The model under review builds one solid part; all positions refer to its coordinate system, in mm. A direction names the side the tool comes from. Give positions to 0.01 mm unless a question says otherwise; leave off trailing zeros. Loops run counter-clockwise (first coordinate to the right, second up) from the corner with the lowest first, then second, coordinate; pieces in that order, holes last. Notation, with made-up numbers: M 17,-33 L 50,-33 A37 cw 50,5 Z; hole C 2,17 d1. An arc over 180 degrees is marked long. One line per item, written item: value. Start each with the question number.
Q1. Mouldability with a two-part tool opening along Y and no side actions: class faces 1 (the face through (-1, 12.5, 3)), 2 (the face through (-56.426, 3.745, 2.958)), 3 (the face through (-32.022, 0.466, 2.958)), 4 (the face through (1, 0, 6)) as released by +Y, released by -Y, zero draft, split by the parting line, or undercut.
Q2. We need section C-C on z = 1. Give the number of separate pieces and of enclosed holes in the cut face, plus the area to 3 significant figures.
Q3. For faces 5 (the face through (16.928, -4.484, 2.958)), 6 (the face through (-37, -7, 3)), 7 (the face through (-33, -10, 3)), list the 3-axis set-ups (+Z, -Z, +X, -X, +Y, -Y) from which the entire face can be reached by the end or side of a thin tool; tool diameter is ignored.
Q4. We need section B-B on y = 0. Write out the cut boundary in (x, z).
Q5. For pin 1 (3.5 mm diameter, centred on x = -35.5, y = -6, fed in from -Z); pin 2 (3 mm diameter, centred on x = -30, z = 3, fed in from -Y); pin 3 (3 mm diameter, centred on y = 5, z = 2.5, fed in from +X), all flat-tipped, find the tip position at first contact; note any pin that passes through.
Q6. We need section D-D on x = -43.5. Write out the cut boundary in (y, z), plus the area to 3 significant figures.
Q7. We need section A-A on x = -5.5. Write out the cut boundary in (y, z).
Q8. To check wall thickness, follow line 1 along X through (y, z) = (5, 5.05); line 2 along X through (y, z) = (-1.75, 0.65); line 3 along Y through (x, z) = (-35.5, 4.75). State the ranges of each line that lie inside material, in increasing order. Write a range as from..to.
```python
from build123d import *

# Parameters (mm, degrees)
SKETCH1_R                                       = 4
SKETCH1_R_2                                     = 1.55
SKETCH1_R_3                                     = 7.5
BOSS_EXTRUDE1_DEPTH                             = 6
CSK_FOR_M5_FLAT_HEAD_MACHINE_SCREW1_D           = 5.5
CSK_FOR_M5_FLAT_HEAD_MACHINE_SCREW1_CSINK_D     = 10.4
CSK_FOR_M5_FLAT_HEAD_MACHINE_SCREW1_CSINK_ANGLE = 90
SKETCH4_R                                       = 1.55
SKETCH4_R_2                                     = 7.5
CUT_EXTRUDE1_DEPTH                              = 59.662168388
SKETCH6_R                                       = 3
CUT_EXTRUDE3_DEPTH                              = 3


with BuildPart() as part:
    # Sketch1 → Boss-Extrude1 (new body)
    with BuildSketch(Plane.XY):
        with BuildLine():
            Line((-44.5, 12.5), (44.5, 12.5))
            ThreePointArc((44.5, 12.5), (57, 0), (44.5, -12.5))
            Line((44.5, -12.5), (-12, -12.5))
            Line((-12, -12.5), (-14.5, -10))
            Line((-14.5, -10), (-52, -10))
            ThreePointArc((-52, -10), (-56.358541226, 3.952847075), (-44.5, 12.5))
        make_face()
        with Locations((10.5, 0)):
            Circle(SKETCH1_R, mode=Mode.SUBTRACT)
        with Locations((15.449747468, 4.949747468)):
            Circle(SKETCH1_R_2, mode=Mode.SUBTRACT)
        with Locations(Location((5.550252532, 4.949747468, 0), (0, 0, 180))):
            Circle(SKETCH1_R_2, mode=Mode.SUBTRACT)
        with Locations((5.550252532, -4.949747468)):
            Circle(SKETCH1_R_2, mode=Mode.SUBTRACT)
        with Locations((15.449747468, -4.949747468)):
            Circle(SKETCH1_R_2, mode=Mode.SUBTRACT)
        with Locations((-33.5, 0)):
            Circle(SKETCH1_R_2, mode=Mode.SUBTRACT)
        with Locations((-19.5, 0)):
            Circle(SKETCH1_R_3, mode=Mode.SUBTRACT)
        with Locations((-5.5, 0)):
            Circle(SKETCH1_R_2, mode=Mode.SUBTRACT)
    extrude(amount=BOSS_EXTRUDE1_DEPTH)

    # CSK for M5 Flat Head Machine Screw1 (through all)
    with Locations(Plane.XY.offset(6)):
        with Locations((44.5, 0)):
            CounterSinkHole(CSK_FOR_M5_FLAT_HEAD_MACHINE_SCREW1_D / 2, CSK_FOR_M5_FLAT_HEAD_MACHINE_SCREW1_CSINK_D / 2, counter_sink_angle=CSK_FOR_M5_FLAT_HEAD_MACHINE_SCREW1_CSINK_ANGLE)

    # Sketch4 → Cut-Extrude1 (cut, through all)
    with BuildSketch(Plane.XY.offset(6)):
        with Locations((-43.5, -6)):
            Circle(SKETCH4_R)
        with Locations((-35.5, -6)):
            Circle(SKETCH4_R)
        with Locations((-19.5, 0)):
            Circle(SKETCH4_R_2)
    extrude(amount=-CUT_EXTRUDE1_DEPTH, mode=Mode.SUBTRACT)

    # Sketch6 → Cut-Extrude3 (cut)
    with BuildSketch(Plane(origin=(0, 0, 0), x_dir=(-1, 0, 0), z_dir=(0, 0, -1))):
        with Locations((43.5, -6)):
            Circle(SKETCH6_R)
        with Locations((35.5, -6)):
            Circle(SKETCH6_R)
    extrude(amount=-CUT_EXTRUDE3_DEPTH, mode=Mode.SUBTRACT)


solid = part.part
```
Solved:
1. face 1: released by +Y
1. face 2: split by the parting line
1. face 3: undercut
1. face 4: zero draft
2. separate pieces: 1
2. enclosed holes: 11
2. area: 2,270 mm2
3. face 5: +Z, -Z
3. face 6: -Z
3. face 7: +Z, -Z, -X, -Y
4. outline: M -57,0 L -35.05,0 L -35.05,6 L -57,6 Z; M -31.95,0 L -27,0 L -27,6 L -31.95,6 Z; M -12,0 L -7.05,0 L -7.05,6 L -12,6 Z; M -3.95,0 L 6.5,0 L 6.5,6 L -3.95,6 Z; M 14.5,0 L 41.75,0 L 41.75,3.55 L 39.3,6 L 14.5,6 Z; M 47.25,0 L 57,0 L 57,6 L 49.7,6 L 47.25,3.55 Z
5. pin 1: z = 3
5. pin 2: y = -10
5. pin 3: x = 56.5
6. outline: M -10,0 L -9,0 L -9,3 L -7.55,3 L -7.55,6 L -10,6 Z; M -4.45,3 L -3,3 L -3,0 L 12.5,0 L 12.5,6 L -4.45,6 Z
6. area: 108 mm2
7. outline: M -12.5,0 L -1.55,0 L -1.55,6 L -12.5,6 Z; M 1.55,0 L 12.5,0 L 12.5,6 L 1.55,6 Z
8. line 1: -55.96..-25.09, -13.91..4, 7.1..13.9, 17..55.96
8. line 2: -56.88..-26.79, -12.21..6.9, 14.1..42.38, 46.62..56.88
8. line 3: -10..-7.55, -4.45..12.5
